```python
from build123d import *

# Parameters (mm, degrees)
F0_W     = 40
F0_H     = 20
F2_DEPTH = 20
F1_R     = 15
F3_DEPTH = 40


with BuildPart() as f2:
    # F0 (on Top) → F2 (new body)
    with BuildSketch(Plane.XY):
        Rectangle(F0_W, F0_H)
    extrude(amount=F2_DEPTH)

    # F1 (on Top) → F3 (join)
    with BuildSketch(Plane.XY):
        with Locations((-31.294566, 0)):
            Circle(F1_R)
        with Locations((31.157609, 0)):
            Circle(F1_R)
    extrude(amount=F3_DEPTH)


solid = f2.part
```
Source: CAD feature listing. Evaluate the final solid. Frame: model axes, mm. A direction names the side the tool comes from. Coordinates: 2 decimals unless noted, no trailing zeros. Loops run counter-clockwise (first coordinate to the right, second up) from the corner with the lowest first, then second, coordinate; pieces in that order, holes last. Notation, with made-up numbers: (86.5, -37) - (103.5, -37) arc R21 ccw to (103.5, -1) - close; hole circle Ø8 at (82.25, 69). An arc over 180 degrees is marked (long way). Answer as CSV lines item,"result".
1. Mould query, pull axis X, two halves, no side actions, for faces 1 (the flat face through (-32, 0, 40)), 2 (the flat face through (0, 10, 10)), 3 (the cylindrical face through (45.465, 4.506, 19.72)). Classes: released by +X, released by -X, zero draft, split by the parting line, or undercut.
Established:
face 1,"zero draft"
face 2,"undercut"
face 3,"undercut"
2. Section A-A (z = 31.5). Return loops of the section in (x, y), then the cut area to 3 significant figures.
Established:
outline,"circle Ø30 at (-31.29, 0); circle Ø30 at (31.16, 0)"
area,"1,410 mm2"
3. Section B-B (y = 0). Return loops of the section in (x, z), then the cut area to 3 significant figures.
Established:
outline,"(-46.29, 0) - (46.16, 0) - (46.16, 40) - (16.16, 40) - (16.16, 20) - (-16.29, 20) - (-16.29, 40) - (-46.29, 40) - close"
area,"3,050 mm2"
4. Section C-C (z = 13.5). Return loops of the section in (x, y).
Established:
outline,"(-20, -10) - (19.98, -10) arc R15 ccw (long way) to (19.98, 10) - (-20, 10) - (-20, 9.87) arc R15 ccw (long way) to (-20, -9.87) - close"
5. Contact query for flat-ended pins moving along their axis: pin 1 (10 mm diameter, centred on x = -9.5, z = 12.5, fed in from -Y); pin 2 (8 mm diameter, centred on x = 17.5, z = 17.5, fed in from -Y); pin 3 (22 mm diameter, centred on x = -2.5, z = 8, fed in from +Y). Output: stop coordinate, or through.
Established:
pin 1,"stops at y = -10"
pin 2,"stops at y = -11.48"
pin 3,"stops at y = 10"
6. Reachability of faces 4 (the flat face through (0, -10, 10)), 5 (the flat face through (31, 0, 40)) from +Z, -Z, +X, -X, +Y, -Y: full face, straight path, thin tool, end or side. Return the list, or none.
Established:
face 4,"+Z, -Z, -Y"
face 5,"+Z, +X, -X, +Y, -Y"
7. Ray query, line 1 (X direction, y = 0.25, z = 29.5); line 2 (X direction, y = -0.5, z = 21); line 3 (Y direction, x = 8.5, z = 8). Return the intervals inside material, ascending.
Established:
line 1,"x = -46.29 to -16.3, 16.16 to 46.16"
line 2,"x = -46.29 to -16.3, 16.17 to 46.15"
line 3,"y = -10 to 10"
8. Section D-D (x = -10.5). Return loops of the section in (y, z).
Established:
outline,"(-10, 0) - (10, 0) - (10, 20) - (-10, 20) - close"
